Verification items for this drawing (mm, ordinates from the low corner). A direction names the side the tool comes from. Round coordinates to 2 decimals unless told otherwise and drop trailing zeros. Loops run counter-clockwise (first coordinate to the right, second up) from the corner with the lowest first, then second, coordinate; pieces in that order, holes last. Notation, with made-up numbers: (44.5, 82) -> (79.5, 82) arc R30 ccw to (79.5, 105) -> close; hole circle Ø1 at (85.5, 19). An arc over 180 degrees is marked (long way). One line per item, written item: value. Start each with the question number.
1. Cross-section at B-B on y = 44. Record the cut outline in (x, z) (1 decimal).
2. Set-up check for the marked faces 4, 5 and 6: record each of +Z, -Z, +X, -X, +Y, -Y from which the full face is reachable in a straight line by a thin tool's end or side.
3. Release check for a two-part mould opening along Y. For the marked faces 1, 2 and 3 record: +Y half, -Y half, draft (parallel to the pull), parting line (faces both ways), or undercut.
4. Cross-section at A-A on z = 5. Count the separate pieces of the cut face and the enclosed holes in it.
5. Material ranges on L1, parallel to X at y = 22.5, z = 1.25 (1 decimal); L2, parallel to Y at x = 36, z = 1.5 (1 decimal); L3, parallel to X at y = 32, z = 5.75 (1 decimal), recorded low to high.
6. Go/stop test with flat-tipped pins: pin 1 (18 mm diameter, centred on x = 76.95, y = 25.75, fed in from -Z); pin 2 (1 mm diameter, centred on x = 25.5, z = 3.5, fed in from -Y) (1 decimal); pin 3 (2 mm diameter, centred on x = 30, z = 2.5, fed in from +Y); pin 4 (1.2 mm diameter, centred on x = 61.5, z = 4.5, fed in from -Y). Record where each tip stops, or that it passes through.
7. Cross-section at C-C on y = 35.5. Record the cut outline in (x, z) (1 decimal).
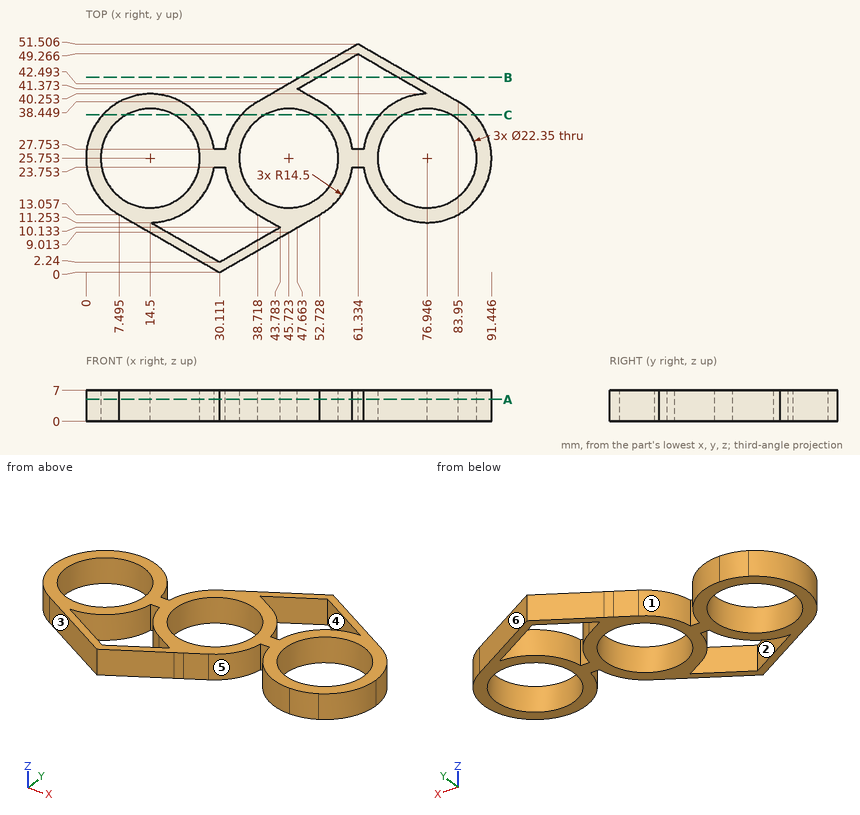
Taken from the geometry:
1. outline: (48.3, 0) -> (52.2, 0) -> (52.2, 7) -> (48.3, 7) -> close; (70.5, 0) -> (74.3, 0) -> (74.3, 7) -> (70.5, 7) -> close
2. face 4: +Z, -Z
2. face 5: +Z, -Z, -Y
2. face 6: +Z, -Z, +X, +Y
3. face 1: +Y half
3. face 2: undercut
3. face 3: -Y half
4. separate pieces: 1
4. enclosed holes: 5
5. L1: x = 0.4 to 3.8, 25.2 to 28.6, 31.6 to 35, 56.4 to 59.9, 62.8 to 66.3, 87.6 to 91.1
5. L2: y = 3.4 to 5.6, 15 to 20.2, 31.3 to 36.5
5. L3: x = 1.4 to 5.2, 23.8 to 27.6, 32.6 to 36.5, 55 to 58.8, 63.9 to 67.7, 86.2 to 90
6. pin 1: passes through
6. pin 2: stops at y = 2.4
6. pin 3: stops at y = 27.75
6. pin 4: stops at y = 23.75
7. outline: (3.8, 0) -> (9, 0) -> (9, 7) -> (3.8, 7) -> close; (20, 0) -> (25.2, 0) -> (25.2, 7) -> (20, 7) -> close; (35, 0) -> (40.3, 0) -> (40.3, 7) -> (35, 7) -> close; (51.2, 0) -> (56.5, 0) -> (56.5, 7) -> (51.2, 7) -> close; (66.2, 0) -> (71.5, 0) -> (71.5, 7) -> (66.2, 7) -> close; (82.4, 0) -> (87.7, 0) -> (87.7, 7) -> (82.4, 7) -> close
